Autodesk Inventor part; units mm, degrees
ref_plane "YZ Plane" through (0, 0, 0) normal (1, 0, 0) x (0, 1, 0)
ref_plane "XZ Plane" through (0, 0, 0) normal (0, 1, 0) x (-1, 0, 0)
ref_plane "XY Plane" through (0, 0, 0) normal (0, 0, 1) x (1, 0, 0)
sketch "Sketch1" plane through (0, 0, 0) normal (0, 0, 1) x (1, 0, 0)
  circle A0 centre (0, 0) radius 20.5
  dimension "d0" = 41
extrude "Extrusion1" add sketch "Sketch1" along normal blind 3
sketch "Sketch2" plane through (0, 0, 3) normal (0, 0, 1) x (1, 0, 0)
  circle A0 centre (0, 0) radius 20.5
  circle A1 centre (0, 0) radius 14.5
  dimension "d3" = 29
extrude "Extrusion2" add sketch "Sketch2" along normal blind 3 contours A1
sketch "Sketch3" plane through (0, 0, 0) normal (0, 0, -1) x (-1, 0, 0)
  circle A0 centre (0, 0) radius 20.5
  circle A1 centre (0, 0) radius 14.5
  dimension "d6" = 29
extrude "Extrusion3" add sketch "Sketch3" along normal blind 2 contours A1
sketch "Sketch4" plane through (0, 0, 3) normal (0, 0, 1) x (1, 0, 0)
  circle A0 centre (0, 0) radius 14.5
  circle A1 centre (0, 0) radius 20.5
  circle A2 centre (0, 0) radius 17.5
  circle A3 centre (0, 17.5) radius 1.5
  circle A4 centre (-12.3744, 12.3744) radius 1.5
  circle A5 centre (-17.5, 0) radius 1.5
  circle A6 centre (-12.3744, -12.3744) radius 1.5
  circle A7 centre (0, -17.5) radius 1.5
  circle A8 centre (12.3744, -12.3744) radius 1.5
  circle A9 centre (17.5, 0) radius 1.5
  circle A10 centre (12.3744, 12.3744) radius 1.5
  dimension "d9" = 35
  dimension "d10" = 3
  dimension "d13" = 360
extrude "Extrusion4" cut sketch "Sketch4" against normal through all contours A2 A9 | A2 A9 | A10 A2 | A2 A10 | A8 A2 | A2 A8 | A3 A2 | A2 A3 | A7 A2 | A2 A7 | A4 A2 | A2 A4 | A6 A2 | A2 A6 | A5 A2 | A2 A5
properties part number "07 CYLINDER FRONT COVER" material "Steel AISI 1020 107 HR"
For this review, take the finished solid that the model builds, in its own axes (mm). A direction names the side the tool comes from. Give positions to 0.01 mm unless a question says otherwise; leave off trailing zeros. Order: outer loops, then holes, each group sorted by start corner. A loop starts at its lowest first (then second) coordinate and runs counter-clockwise, first axis right, second up.
1) Wall thickness on line 1 (Y direction, x = -13, z = 1.5); line 2 (X direction, y = 17.5, z = 2.15); line 3 (Z direction, x = 15.5, y = 12.5): over which ranges is each line inside the solid? List them lowest first.
2) Take a section at B-B (x = -13). Give the boundary of the cut face in (y, z), then the cut area to 3 significant figures.
3) Insertion check: pin 1 (4 mm diameter, centred on x = 0, y = -17.5, fed in from +Z); pin 2 (2.5 mm diameter, centred on x = 12.37, y = 12.37, fed in from -Z); pin 3 (1.5 mm diameter, centred on x = -9, z = -1, fed in from -Y); pin 4 (1.5 mm diameter, centred on y = 2, z = -0.5, fed in from +X). Each pin has a flat end and moves straight along its axis. Give the tip position at first contact, or say it passes through.
4) Take a section at C-C (y = -17.5). Give the boundary of the cut face in (x, z).
5) Take a section at A-A (y = 0). Give the boundary of the cut face in (x, z), then the cut area to 3 significant figures.
6) For faces 1 (the face through (13.805, -11.924, 1.521)), 2 (the face through (-6, 14, 0)), 3 (the face through (6.691, 12.864, 4.479)), list the 3-axis set-ups (+Z, -Z, +X, -X, +Y, -Y) from which the entire face can be reached by the end or side of a thin tool; tool diameter is ignored.
7) The part is to be moulded in two halves that separate along X. For faces 4 (the face through (0, 0, -2)), 5 (the face through (-4.444, 20.013, 1.479)), 6 (the face through (0, -16, 2)), say which applies: released by +X, released by -X, zero draft, split by the parting line, or undercut.
8) Take a section at D-D (x = 17). Give the boundary of the cut face in (y, z), then the cut area to 3 significant figures.
Derived:
1. line 1: y = -15.85 to -13.74, -11.01 to 11.01, 13.74 to 15.85
1. line 2: x = -10.68 to -1.5, 1.5 to 10.68
1. line 3: z = 0 to 3
2. outline: (-15.85, 0) - (-13.74, 0) - (-13.74, 3) - (-15.85, 3) - close; (-11.01, 0) - (-6.42, 0) - (-6.42, -2) - (6.42, -2) - (6.42, 0) - (11.01, 0) - (11.01, 3) - (6.42, 3) - (6.42, 6) - (-6.42, 6) - (-6.42, 3) - (-11.01, 3) - close; (13.74, 0) - (15.85, 0) - (15.85, 3) - (13.74, 3) - close
2. area: 143 mm2
3. pin 1: stops at z = 3
3. pin 2: passes through
3. pin 3: stops at y = -11.92
3. pin 4: stops at x = 20.45
4. outline: (-10.68, 0) - (-1.5, 0) - (-1.5, 3) - (-10.68, 3) - close; (1.5, 0) - (10.68, 0) - (10.68, 3) - (1.5, 3) - close
5. outline: (-20.5, 0) - (-19, 0) - (-19, 3) - (-20.5, 3) - close; (-16, 0) - (-14.5, 0) - (-14.5, -2) - (14.5, -2) - (14.5, 0) - (16, 0) - (16, 3) - (14.5, 3) - (14.5, 6) - (-14.5, 6) - (-14.5, 3) - (-16, 3) - close; (19, 0) - (20.5, 0) - (20.5, 3) - (19, 3) - close
5. area: 250 mm2
6. face 1: +Z, -Z
6. face 2: -Z
6. face 3: +Z
7. face 4: zero draft
7. face 5: split by the parting line
7. face 6: undercut
8. outline: (-11.46, 0) - (-1.41, 0) - (-1.41, 3) - (-11.46, 3) - close; (1.41, 0) - (11.46, 0) - (11.46, 3) - (1.41, 3) - close
8. area: 60.3 mm2
